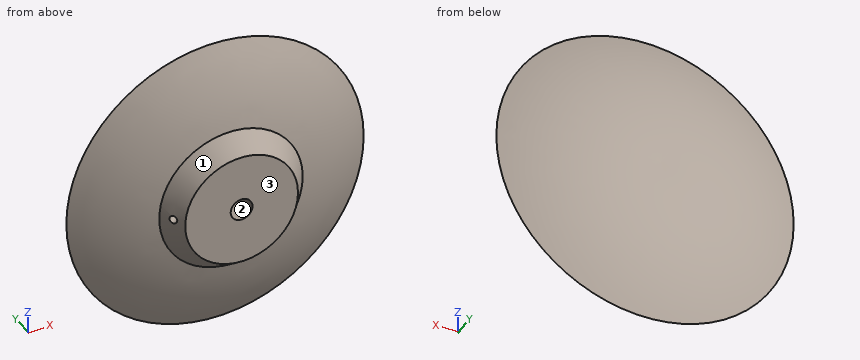
```python
from build123d import *

# Parameters (mm, degrees)
F_5_8_11_TAPPED_HOLE1_D            = 13.49248
F_5_8_11_TAPPED_HOLE1_DEPTH        = 19.05
F_5_8_11_TAPPED_HOLE1_TIP          = 4.053549943
F_3_16_0_1875_DIAMETER_HOLE1_D     = 4.7625
F_3_16_0_1875_DIAMETER_HOLE1_DEPTH = 12.7
F_3_16_0_1875_DIAMETER_HOLE1_TIP   = 1.430799349


with BuildPart() as part:
    # Sketch1 → Revolve1 (revolve)
    with BuildSketch(Plane.XY):
        with BuildLine():
            Line((0, 0), (34.925, 0))
            Line((34.925, 0), (44.45, 12.7))
            add(Edge.make_bspline(
                [(44.45, 12.7), (69.750610432, 18.159935057), (92.075, 31.75)],
                knots=[0, 0, 0, 1, 1, 1], degree=2))
            add(Edge.make_bspline(
                [(92.075, 31.75), (49.236918404, 53.116611797), (0, 50.8)],
                knots=[0, 0, 0, 1, 1, 1], degree=2))
            Line((0, 50.8), (0, 31.75))
            Line((0, 31.75), (0, 12.7))
            Line((0, 12.7), (0, 0))
        make_face()
    revolve(axis=Axis((0, 31.75, 0), (0, 1, 0)))

    # 5/8-11 Tapped Hole1
    with Locations(Plane(origin=(0, 0, 0), x_dir=(-1, 0, 0), z_dir=(0, -1, 0))):
        with Locations((0, 0)):
            Hole(F_5_8_11_TAPPED_HOLE1_D / 2, depth=F_5_8_11_TAPPED_HOLE1_DEPTH)
            with Locations((0, 0, -(F_5_8_11_TAPPED_HOLE1_DEPTH + F_5_8_11_TAPPED_HOLE1_TIP / 2))):  # 118° drill point
                Cone(0, F_5_8_11_TAPPED_HOLE1_D / 2, F_5_8_11_TAPPED_HOLE1_TIP, mode=Mode.SUBTRACT)

    # 3/16 (0.1875) Diameter Hole1
    with Locations(Plane(origin=(-39.246742436, 5.838388433, 2.116889387), x_dir=(0.600557743, -0.799581389, 0), z_dir=(-0.798838811, -0.6, 0.043087739))):
        with Locations((0, 0)):
            Hole(F_3_16_0_1875_DIAMETER_HOLE1_D / 2, depth=F_3_16_0_1875_DIAMETER_HOLE1_DEPTH)
            with Locations((0, 0, -(F_3_16_0_1875_DIAMETER_HOLE1_DEPTH + F_3_16_0_1875_DIAMETER_HOLE1_TIP / 2))):  # 118° drill point
                Cone(0, F_3_16_0_1875_DIAMETER_HOLE1_D / 2, F_3_16_0_1875_DIAMETER_HOLE1_TIP, mode=Mode.SUBTRACT)


solid = part.part
```
Geometry check sheet. Reference: the model listing, model coordinates, mm. Face numbers are marked on the shaded views. Coordinates: 2 decimals unless noted, no trailing zeros.
Item 1: Go/stop test with flat-tipped pins: pin 1 Ø1 at (x, z) = (30.5, 28.5) entering from -Y; pin 2 Ø1 at (x, z) = (23.5, 70.5) entering from +Y; pin 3 Ø12 at (x, z) = (-45, 32) entering from +Y. Record where each tip stops, or that it passes through.
Item 2: Release check for a two-part mould opening along X. For the marked faces 1, 2 and 3 record: released by +X, released by -X, zero draft, split by the parting line, or undercut.
Item 3: Thickness scan on line 1 (Z direction, x = 0, y = 8.5); line 2 (Y direction, x = -9.5, z = 7.5); line 3 (Z direction, x = 0, y = 8) (3 decimals). Record the ranges inside material, lowest first.
Check result:
1. pin 1: stops at y = 8.42
1. pin 2: stops at y = 39.67
1. pin 3: stops at y = 46.86
2. face 1: split by the parting line
2. face 2: undercut
2. face 3: zero draft
3. line 1: z = -41.3 to -6.75, 6.75 to 41.3
3. line 2: y = 0 to 51.01
3. line 3: z = -40.925 to -6.746, 6.746 to 40.925
